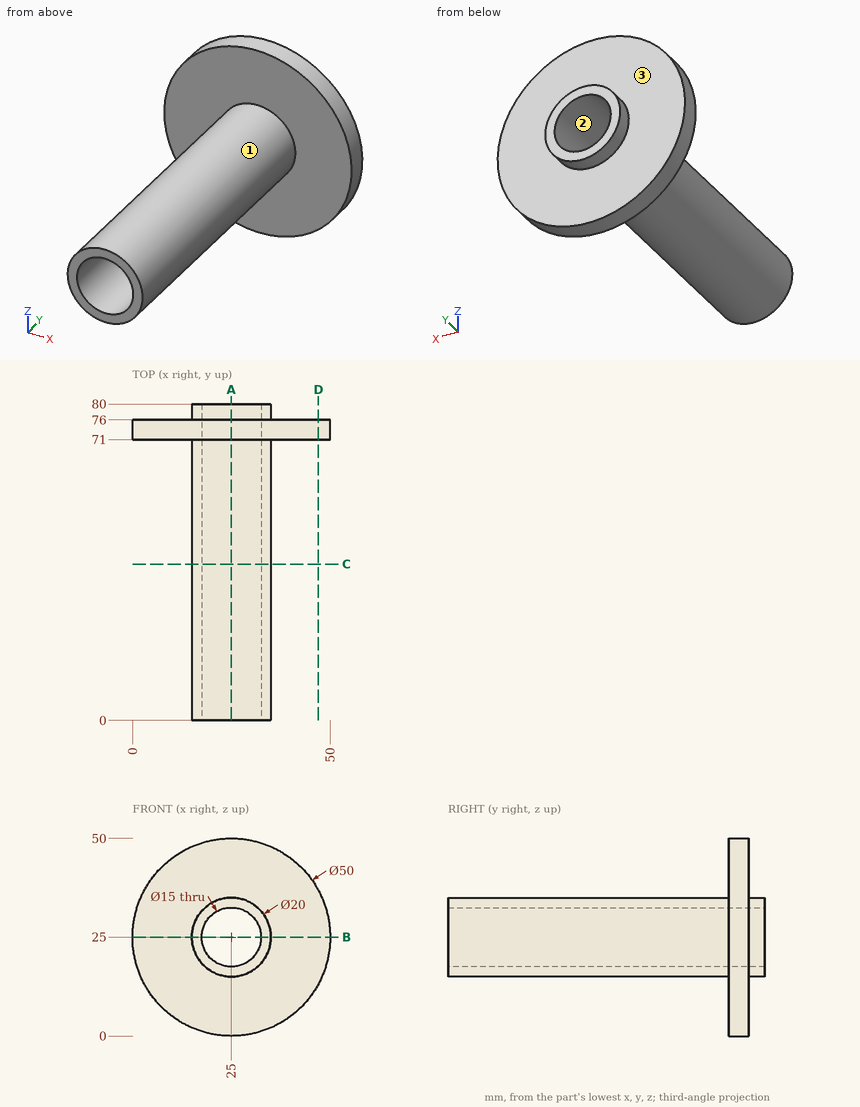
Check sheet for the drawn part. Datum: minimum x, y, z corner. Units: mm. Give positions to 0.01 mm unless a question says otherwise; leave off trailing zeros. Order: outer loops, then holes, each group sorted by start corner. A loop starts at its lowest first (then second) coordinate and runs counter-clockwise, first axis right, second up. Notation, with made-up numbers: (-31.75, 21.5) - (26.25, 21.5) arc R28 ccw to (26.25, 55.5) - close; hole circle Ø10 at (-6.75, 44.25). An arc over 180 degrees is marked (long way). Answer as a JSON object with one key per item and string values.
(1) Cross-section at D-D (x = 47). Record the cut outline in (y, z), then the cut area to 3 significant figures.
Report:
{"outline": "(71, 13.13) - (76, 13.13) - (76, 36.87) - (71, 36.87) - close", "area": "119 mm^2"}
(2) Cross-section at C-C (y = 39.5). Record the cut outline in (x, z).
Report:
{"outline": "circle Ø20 at (25, 25); hole circle Ø15 at (25, 25)"}
(3) Draft check along Z on the marked faces 1, 2 and 3. Enter one of: released by +Z, released by -Z, zero draft, split by the parting line, or undercut.
Report:
{"face 1": "split by the parting line", "face 2": "undercut", "face 3": "zero draft"}
(4) Material ranges on line 1 (X direction, y = 18, z = 25); line 2 (Z direction, x = 22.5, y = 40.5); line 3 (Y direction, x = 9, z = 37), recorded low to high.
Report:
{"line 1": "15 to 17.5, 32.5 to 35", "line 2": "15.32 to 17.93, 32.07 to 34.68", "line 3": "71 to 76"}
(5) Cross-section at B-B (z = 25). Record the cut outline in (x, y).
Report:
{"outline": "(0, 71) - (15, 71) - (15, 0) - (17.5, 0) - (17.5, 80) - (15, 80) - (15, 76) - (0, 76) - close; (32.5, 0) - (35, 0) - (35, 71) - (50, 71) - (50, 76) - (35, 76) - (35, 80) - (32.5, 80) - close"}
(6) Cross-section at A-A (x = 25). Record the cut outline in (y, z).
Report:
{"outline": "(0, 15) - (71, 15) - (71, 0) - (76, 0) - (76, 15) - (80, 15) - (80, 17.5) - (0, 17.5) - close; (0, 32.5) - (80, 32.5) - (80, 35) - (76, 35) - (76, 50) - (71, 50) - (71, 35) - (0, 35) - close"}
(7) Depth check by flat-ended pin: pin 1 Ø15 at (x, z) = (28, 23.5) entering from +Y; pin 2 Ø1.5 at (x, z) = (27, 9.5) entering from +Y; pin 3 Ø5 at (x, y) = (14, 43) entering from +Z; pin 4 Ø5 at (x, y) = (13.5, 49) entering from +Z. Enter the tip coordinate at first touch or a pass-through.
Report:
{"pin 1": "y = 80", "pin 2": "y = 76", "pin 3": "z = 30.27", "pin 4": "z = 29.36"}
